Part model, mm, in its own coordinate system. Face numbers are marked on the shaded views. Round coordinates to 2 decimals unless told otherwise and drop trailing zeros. Order: outer loops, then holes, each group sorted by start corner. A loop starts at its lowest first (then second) coordinate and runs counter-clockwise, first axis right, second up. Notation, with made-up numbers: (-20.5, 32) - (2.5, 32) arc R19 ccw to (2.5, 69) - close; hole circle Ø3 at (34, 45.25). An arc over 180 degrees is marked (long way). Return JSON: item names as keys, results as strings. Group by question number.
Item 1: Probe probe 1 along X at (y, z) = (1, 6); probe 2 along Z at (x, y) = (10, 4); probe 3 along X at (y, z) = (3.5, 10). List the from-to ranges inside material, lowest first.
Item 2: Saw through at D-D on z = -6. List the corners of the cut face in (x, y), and give its area (4 significant figures).
Item 3: Drop flat-ended pins along their axis: pin 1 (1 mm diameter, centred on y = 1, z = 5.5, fed in from +X); pin 2 (1.5 mm diameter, centred on x = 8.5, y = 3.5, fed in from +Z). Give the stop position or say it passes through.
Item 4: Saw through at B-B on z = 5.5. List the corners of the cut face in (x, y).
Item 5: Saw through at A-A on x = 0. List the corners of the cut face in (y, z) (3 decimals).
Item 6: Two-plate mould, pull along Z, no slides. Class the marked faces 1, 2, 3 and 4: released by +Z, released by -Z, zero draft, split by the parting line, or undercut.
Item 7: Saw through at C-C on x = 9.75. List the corners of the cut face in (y, z).
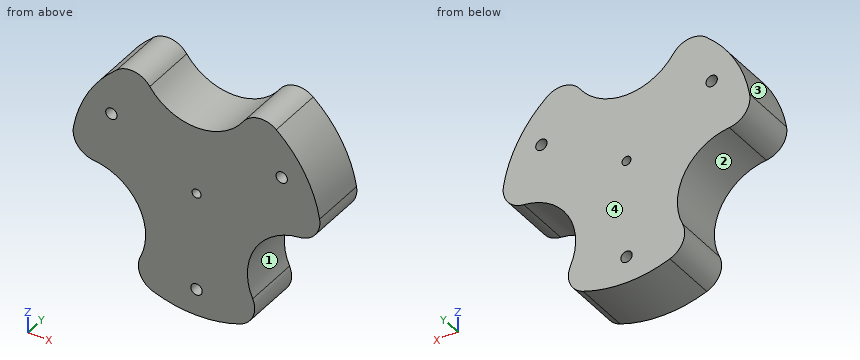
```python
from build123d import *

# Parameters (mm, degrees)
SKETCH1_R                       = 13.97
BOSS_EXTRUDE1_DEPTH             = 6.35
SKETCH2_R                       = 0.635
CUT_EXTRUDE1_DEPTH              = 7.35
CIRPATTERN1_COUNT               = 3
SKETCH4_R                       = 6.406839675
CUT_EXTRUDE3_DEPTH              = 7.35
CIRPATTERN2_COUNT               = 3
FILLET1_R                       = 2.54
F_1_0MM_PRESS_DOWEL_HOLE1_D     = 1
F_1_0MM_PRESS_DOWEL_HOLE1_DEPTH = 24.892
F_1_0MM_PRESS_DOWEL_HOLE1_TIP   = 0.30043031


with BuildPart() as part:
    # Sketch1 → Boss-Extrude1 (new body)
    with BuildSketch(Plane(origin=(0, 0, 0), x_dir=(1, 0, 0), z_dir=(0, 1, 0))):
        Circle(SKETCH1_R)
    extrude(amount=BOSS_EXTRUDE1_DEPTH)

    # Sketch2 → Cut-Extrude1 (cut, through all)
    with BuildSketch(Plane(origin=(0, 6.35, 0), x_dir=(1, 0, 0), z_dir=(0, 1, 0))):
        with Locations((0, 11)):
            Circle(SKETCH2_R)
    cut_extrude1 = extrude(amount=-CUT_EXTRUDE1_DEPTH, mode=Mode.SUBTRACT)

    # CirPattern1: Cut-Extrude1 ×3 about axis
    cirpattern1_axis = Axis((0, 0, 0), (0, 1, 0))
    for i in range(1, CIRPATTERN1_COUNT):
        add(cut_extrude1.rotate(cirpattern1_axis, i * 360 / CIRPATTERN1_COUNT), mode=Mode.SUBTRACT)

    # Sketch4 → Cut-Extrude3 (cut, through all)
    with BuildSketch(Plane(origin=(0, 6.35, 0), x_dir=(1, 0, 0), z_dir=(0, 1, 0))):
        with Locations((0, -13.97)):
            Circle(SKETCH4_R)
    cut_extrude3 = extrude(amount=-CUT_EXTRUDE3_DEPTH, mode=Mode.SUBTRACT)

    # CirPattern2: Cut-Extrude3 ×3 about axis
    cirpattern2_axis = Axis((0, 0, 0), (0, 1, 0))
    for i in range(1, CIRPATTERN2_COUNT):
        add(cut_extrude3.rotate(cirpattern2_axis, i * 360 / CIRPATTERN2_COUNT), mode=Mode.SUBTRACT)

    # Fillet1
    fillet1_edges = [part.edges().sort_by_distance(p)[0] for p in [
        (-6.236123867, 3.175, 12.500866334),
        (6.236123867, 3.175, 12.500866334),
        (-7.708005881, 3.175, -11.651074857),
        (-13.944129749, 3.175, -0.849791477),
        (13.944129749, 3.175, -0.849791477),
        (7.708005881, 3.175, -11.651074857),
    ]]
    fillet(fillet1_edges, radius=FILLET1_R)

    # 1.0mm Press Dowel Hole1
    with Locations(Plane(origin=(0, 6.35, 0), x_dir=(1, 0, 0), z_dir=(0, 1, 0))):
        with Locations((0, 0)):
            Hole(F_1_0MM_PRESS_DOWEL_HOLE1_D / 2, depth=F_1_0MM_PRESS_DOWEL_HOLE1_DEPTH)
            with Locations((0, 0, -(F_1_0MM_PRESS_DOWEL_HOLE1_DEPTH + F_1_0MM_PRESS_DOWEL_HOLE1_TIP / 2))):  # 118° drill point
                Cone(0, F_1_0MM_PRESS_DOWEL_HOLE1_D / 2, F_1_0MM_PRESS_DOWEL_HOLE1_TIP, mode=Mode.SUBTRACT)


solid = part.part
```
Filled in:
{
 "1": {"probe 1": "x = -12.62 to -9.92, -9.13 to 9.13, 9.92 to 12.62", "probe 2": "z = -0.93 to 5.08, 5.92 to 9.76", "probe 3": "x = -9.76 to -5.03, 5.03 to 9.76"},
 "2": {"outline": "(-5.77, 0) - (5.77, 0) - (5.77, 6.35) - (-5.77, 6.35) - close", "area": "73.25 mm^2"},
 "3": {"pin 1": "stops at x = 13.04", "pin 2": "stops at z = 11.3"},
 "4": {"outline": "(-12.84, 0) - (-10.16, 0) - (-10.16, 6.35) - (-12.84, 6.35) - close; (-8.89, 0) - (8.89, 0) - (8.89, 6.35) - (-8.89, 6.35) - close; (10.16, 0) - (12.84, 0) - (12.84, 6.35) - (10.16, 6.35) - close"},
 "5": {"outline": "(0, -13.97) - (6.35, -13.97) - (6.35, -11.635) - (0, -11.635) - close; (0, -10.365) - (6.35, -10.365) - (6.35, -0.5) - (0, -0.5) - close; (0, 0.5) - (6.35, 0.5) - (6.35, 7.563) - (0, 7.563) - close"},
 "6": {"face 1": "undercut", "face 2": "undercut", "face 3": "released by +Z", "face 4": "zero draft"},
 "7": {"outline": "(0, -1.02) - (6.35, -1.02) - (6.35, 4.91) - (0, 4.91) - close; (0, 6.09) - (6.35, 6.09) - (6.35, 10) - (0, 10) - close"}
}
